Study the drawing (mm; zero at the part's minimum x, y, z) and answer. Round coordinates to 2 decimals unless told otherwise and drop trailing zeros. Order: outer loops, then holes, each group sorted by start corner. A loop starts at its lowest first (then second) coordinate and runs counter-clockwise, first axis right, second up. Notation, with made-up numbers: (83, 27) - (105, 27) arc R18 cw to (105, 41) - close; hole circle Ø9 at (-36.5, 29.5). An arc over 180 degrees is marked (long way). Put each result on its own line as item: value.
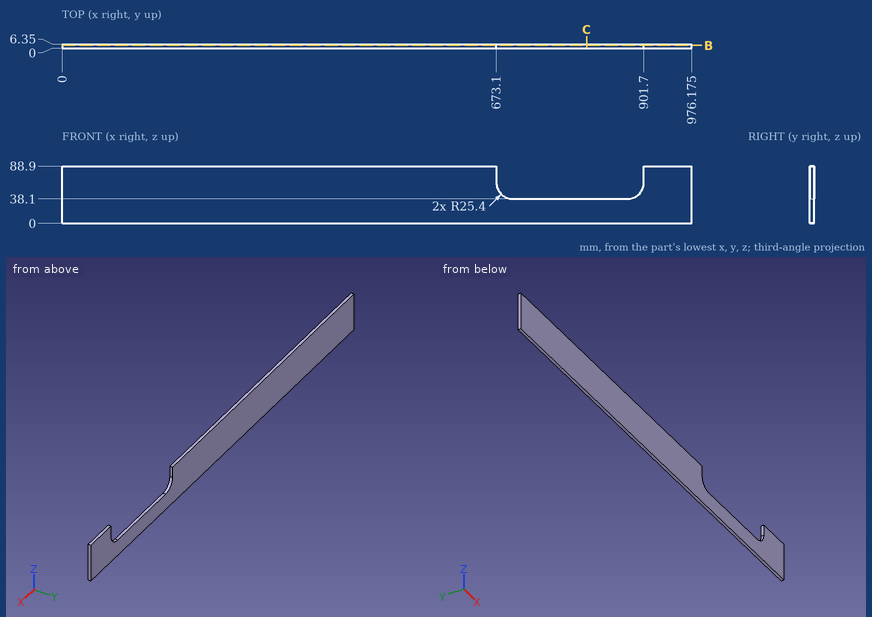
1) A cutting plane is placed at C-C on x = 813. Write down the section's boundary in (y, z), then the cut area to 3 significant figures.
Findings below:
outline: (0, 0) - (6.35, 0) - (6.35, 38.1) - (0, 38.1) - close
area: 242 mm2
2) A cutting plane is placed at B-B on y = 4.25. Write down the section's boundary in (x, z) (1 decimal), then the cut area to 3 significant figures.
Findings below:
outline: (0, 0) - (976.2, 0) - (976.2, 88.9) - (901.7, 88.9) - (901.7, 63.5) arc R25.4 cw to (876.3, 38.1) - (698.5, 38.1) arc R25.4 cw to (673.1, 63.5) - (673.1, 88.9) - (0, 88.9) - close
area: 75,400 mm2
3) Given pin 1 Ø1.9 at (y, z) = (2.5, 71) entering from -X, flat-ended and moving along its own axis, determine where the tip first touches the part or whether it passes through.
Findings below:
pin 1: stops at x = 0
4) Straight lines are drawn through the part: L1, parallel to X at y = 3.5, z = 64 (1 decimal); L2, parallel to X at y = 2.5, z = 49 (1 decimal); L3, parallel to Z at x = 803, y = 6. For each, find the intervals that lie inside material, in ascending order. Write a range as from..to.
Findings below:
L1: x = 0..673.1, 901.7..976.2
L2: x = 0..677.6, 897.2..976.2
L3: z = 0..38.1
